```python
from build123d import *

# Parameters (mm, degrees)
HEX_2_DEPTH = 2.2098


with BuildPart() as part:
    # BodySke → BaseBody (revolve)
    with BuildSketch(Plane.XY, mode=Mode.PRIVATE) as basebody_sk:
        with BuildLine():
            Line((28.7528, 0), (28.7528, 2.41935))
            Line((28.7528, 2.41935), (27.99715, 3.175))
            Line((27.99715, 3.175), (3.3528, 3.175))
            Line((3.3528, 3.175), (3.3528, 5.5499))
            Line((3.3528, 5.5499), (2.5654, 5.5499))
            ThreePointArc((2.5654, 5.5499), (1.073764503, 4.355582759), (0, 2.77495))
            Line((0, 2.77495), (0, 0))
            Line((0, 0), (28.7528, 0))
        make_face()
    revolve(basebody_sk.sketch.rotate(Axis((0, 0, 0), (1, 0, 0)), 90), axis=Axis((0, 0, 0), (1, 0, 0)))

    # Sketch2 → PreBroach (revolve, cut)
    with BuildSketch(Plane.XY, mode=Mode.PRIVATE) as prebroach_sk:
        Polygon((0, 1.9812), (2.2098, 1.9812), (3.353646353, 0), (0, 0), align=None)
    revolve(prebroach_sk.sketch.rotate(Axis((0, 0, 0), (1, 0, 0)), 90), axis=Axis((0, 0, 0), (1, 0, 0)), mode=Mode.SUBTRACT)

    # Sketch3 → Hex 2 (cut)
    with BuildSketch(Plane(origin=(0, 0, 0), x_dir=(0, 0, -1), z_dir=(1, 0, 0))):
        Polygon((-1.9812, -1.143846353), (-1.9812, 1.143846353), (0, 2.287692707), (1.9812, 1.143846353), (1.9812, -1.143846353), (0, -2.287692707), align=None)
    extrude(amount=HEX_2_DEPTH, mode=Mode.SUBTRACT)


solid = part.part
```
The listing builds one solid part. Answer for the finished solid, in the listing's coordinates (mm). A direction names the side the tool comes from. Round coordinates to 2 decimals unless told otherwise and drop trailing zeros. Write each loop counter-clockwise with the first axis right and the second up, starting at its lowest first coordinate (ties: lowest second). Pieces come first, ordered by that corner, then holes. Notation, with made-up numbers: (-27.75, 2) -> (-1.75, 2) arc R12 cw to (-1.75, 24) -> close; hole circle Ø3 at (16.5, 34.5). An arc over 180 degrees is marked (long way). Answer as a JSON object with one key per item and string values. Group by question number.
Q1. Section C-C (y = 5.25) is taken. Write down the section's boundary in (x, z), plus the area to 3 significant figures.
Q2. Each of these flat-tipped pins is pushed along its axis until it touches: pin 1 Ø0.5 at (y, z) = (-1, 1.5) entering from -X; pin 2 Ø5 at (x, z) = (12.5, 2.5) entering from +Y (3 decimals); pin 3 Ø3 at (x, z) = (9, -0.5) entering from -Y (3 decimals). Where does it stop, or does it pass through?
Q3. Section B-B (z = -4.5) is taken. Write down the section's boundary in (x, y), plus the area to 3 significant figures.
Q4. Determine the mould class of faces 1 (the face through (1.09, 1.71, 1)), 2 (the face through (15.5, 1.93, -2.52)), 3 (the face through (0, -2, 1)) for opening direction Z: pulls with the +Z half, pulls with the -Z half, needs draft (parallel to the pull), parting line crosses it, or undercut.
Q5. Section A-A (x = 18) is taken. Write down the section's boundary in (y, z) (3 decimals).
Q6. Which of the six approach directions +Z, -Z, +X, -X, +Y, -Y give full straight-line access (tool end or side, diameter ignored) to faces 4 (the face through (3.353, 2.4, -2.4)), 5 (the face through (1, 0, 1.981)), 6 (the face through (2.954, 4.924, 2.561))?
Q7. Straight lines are drawn through the part: line 1 along Y through (x, z) = (12.75, 0) (3 decimals); line 2 along X through (y, z) = (3.75, -3.25); line 3 along Y through (x, z) = (1.5, -0.5). For each, find the intervals that lie inside material, in ascending order.
Check values:
{
 "1": {"outline": "(2.57, -1.8) -> (3.35, -1.8) -> (3.35, 1.8) -> (2.57, 1.8) arc R3.69 ccw to start", "area": "3.97 mm^2"},
 "2": {"pin 1": "x = 2.21", "pin 2": "y = 3.175", "pin 3": "y = -3.175"},
 "3": {"outline": "(2.57, -3.25) -> (3.35, -3.25) -> (3.35, 3.25) -> (2.57, 3.25) arc R4.57 ccw to start", "area": "11.2 mm^2"},
 "4": {"face 1": "undercut", "face 2": "parting line crosses it", "face 3": "needs draft"},
 "5": {"outline": "circle Ø6.35 at (0, 0)"},
 "6": {"face 4": "+X", "face 5": "-X", "face 6": "+X, -X"},
 "7": {"line 1": "-3.175 to 3.175", "line 2": "1.72 to 3.35", "line 3": "-4.75 to -2, 2 to 4.75"}
}
